Work out the finished part from the listing and answer in its coordinate system (mm). Coordinates: 2 decimals unless noted, no trailing zeros. Loops run counter-clockwise (first coordinate to the right, second up) from the corner with the lowest first, then second, coordinate; pieces in that order, holes last. Notation, with made-up numbers: (41, 48.25) -> (86, 48.25) arc R35 cw to (86, 81.25) -> close; hole circle Ø5 at (60.5, -19). An arc over 180 degrees is marked (long way). Answer as CSV lines item,"result".
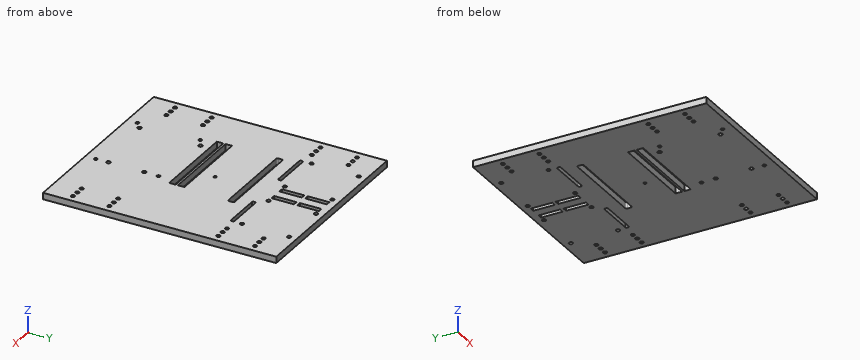
```python
from build123d import *

# Parameters (mm, degrees)
F0_R     = 1.494301
F0_R_2   = 1.356788
F0_R_3   = 1.5875
F0_W     = 66.04
F0_H     = 5.08
F0_W_2   = 3.491225
F0_H_2   = 17.486991
F0_H_3   = 16.910404
F0_R_4   = 1.133922
F1_DEPTH = 5.0038


with BuildPart() as f1:
    # F0 (on Top) → F1 (new body)
    with BuildSketch(Plane.XY):
        Polygon((70.456985, 90.965845), (-70.456985, 90.965845), (-76.806985, 90.965845), (-76.806985, 84.615845), (-76.806985, -84.615845), (-76.806985, -90.965845), (-70.456985, -90.965845), (70.456985, -90.965845), (76.806985, -90.965845), (76.806985, -84.615845), (76.806985, 84.615845), (76.806985, 90.965845), align=None)
        with Locations((-70.824079, -70.982955)):
            Circle(F0_R, mode=Mode.SUBTRACT)
        with Locations((-64.820901, -70.966512)):
            Circle(F0_R, mode=Mode.SUBTRACT)
        with Locations((-58.837254, -70.966512)):
            Circle(F0_R, mode=Mode.SUBTRACT)
        with Locations((-39.865345, -82.879322)):
            Circle(F0_R_2, mode=Mode.SUBTRACT)
        with Locations((-34.309838, -78.185227)):
            Circle(F0_R_3, mode=Mode.SUBTRACT)
        with Locations((-70.834705, -42.482955)):
            Circle(F0_R, mode=Mode.SUBTRACT)
        with Locations((-64.831526, -42.467712)):
            Circle(F0_R, mode=Mode.SUBTRACT)
        with Locations((-58.847879, -42.467712)):
            Circle(F0_R, mode=Mode.SUBTRACT)
        with Locations((-39.865345, -33.888042)):
            Circle(F0_R_2, mode=Mode.SUBTRACT)
        with Locations((-33.039838, -29.925227)):
            Circle(F0_R_3, mode=Mode.SUBTRACT)
        with Locations((-10.337991, -20.430786)):
            Rectangle(F0_W, F0_H, mode=Mode.SUBTRACT)
        with Locations((-10.337991, -13.637)):
            Rectangle(F0_W, F0_H, mode=Mode.SUBTRACT)
        with Locations((18.120408, -82.87932)):
            Circle(F0_R_2, mode=Mode.SUBTRACT)
        with Locations((17.760162, -73.105227)):
            Circle(F0_R_3, mode=Mode.SUBTRACT)
        with Locations((58.837254, -70.966512)):
            Circle(F0_R, mode=Mode.SUBTRACT)
        with Locations((64.820901, -70.966512)):
            Circle(F0_R, mode=Mode.SUBTRACT)
        with Locations((70.824079, -70.982955)):
            Circle(F0_R, mode=Mode.SUBTRACT)
        with Locations((17.760162, -45.165227)):
            Circle(F0_R_3, mode=Mode.SUBTRACT)
        with Locations((18.120408, -33.888042)):
            Circle(F0_R_2, mode=Mode.SUBTRACT)
        with Locations((58.847879, -42.467712)):
            Circle(F0_R, mode=Mode.SUBTRACT)
        with Locations((64.831526, -42.467712)):
            Circle(F0_R, mode=Mode.SUBTRACT)
        with Locations((70.834705, -42.482955)):
            Circle(F0_R, mode=Mode.SUBTRACT)
        with Locations((-70.834705, 42.482955)):
            Circle(F0_R, mode=Mode.SUBTRACT)
        with Locations((-64.831526, 42.467712)):
            Circle(F0_R, mode=Mode.SUBTRACT)
        with Locations((-58.847878, 42.482955)):
            Circle(F0_R, mode=Mode.SUBTRACT)
        with BuildLine():
            ThreePointArc((-48.263557, 40.736089), (-47.935968, 41.52696), (-47.145098, 41.854549))
            Line((-47.145098, 41.854549), (-34.13846, 41.854549))
            Line((-34.13846, 41.854549), (-31.515838, 41.854549))
            Line((-31.515838, 41.854549), (-18.5092, 41.854549))
            ThreePointArc((-18.5092, 41.854549), (-17.718329, 41.52696), (-17.39074, 40.736089))
            Line((-17.39074, 40.736089), (-17.39074, 40.22988))
            ThreePointArc((-17.39074, 40.22988), (-17.718329, 39.43901), (-18.5092, 39.111421))
            Line((-18.5092, 39.111421), (-31.515838, 39.111421))
            Line((-31.515838, 39.111421), (-34.13846, 39.111421))
            Line((-34.13846, 39.111421), (-47.145098, 39.111421))
            ThreePointArc((-47.145098, 39.111421), (-47.935968, 39.43901), (-48.263557, 40.22988))
            Line((-48.263557, 40.22988), (-48.263557, 40.736089))
        make_face(mode=Mode.SUBTRACT)
        with BuildLine():
            Line((23.800469, 23.877405), (-42.239531, 23.877405))
            ThreePointArc((-42.239531, 23.877405), (-43.030401, 24.204994), (-43.357991, 24.995864))
            Line((-43.357991, 24.995864), (-43.357991, 27.672048))
            ThreePointArc((-43.357991, 27.672048), (-43.030401, 28.462918), (-42.239531, 28.790507))
            Line((-42.239531, 28.790507), (15.032583, 28.790507))
            Line((15.032583, 28.790507), (19.658049, 28.790507))
            Line((19.658049, 28.790507), (23.800469, 28.790507))
            ThreePointArc((23.800469, 28.790507), (24.59134, 28.462918), (24.918929, 27.672048))
            Line((24.918929, 27.672048), (24.918929, 24.995864))
            ThreePointArc((24.918929, 24.995864), (24.59134, 24.204994), (23.800469, 23.877405))
        make_face(mode=Mode.SUBTRACT)
        with Locations((-48.263557, 48.184544)):
            Circle(F0_R, mode=Mode.SUBTRACT)
        with Locations((-70.824079, 70.982955)):
            Circle(F0_R, mode=Mode.SUBTRACT)
        with Locations((-64.820901, 70.966512)):
            Circle(F0_R, mode=Mode.SUBTRACT)
        with Locations((-58.837252, 70.981755)):
            Circle(F0_R, mode=Mode.SUBTRACT)
        with Locations((-48.292145, 85.000329)):
            Circle(F0_R, mode=Mode.SUBTRACT)
        with Locations((-11.321435, 48.135974)):
            Circle(F0_R, mode=Mode.SUBTRACT)
        with Locations((-5.441815, 56.879467)):
            Rectangle(F0_W_2, F0_H_2, mode=Mode.SUBTRACT)
        with Locations((-5.441815, 76.696746)):
            Rectangle(F0_W_2, F0_H_3, mode=Mode.SUBTRACT)
        with Locations((-11.321435, 85.151948)):
            Circle(F0_R, mode=Mode.SUBTRACT)
        Circle(F0_R_4, mode=Mode.SUBTRACT)
        with BuildLine():
            Line((31.515838, 39.111421), (18.5092, 39.111421))
            ThreePointArc((18.5092, 39.111421), (17.718329, 39.43901), (17.39074, 40.22988))
            Line((17.39074, 40.22988), (17.39074, 40.736089))
            ThreePointArc((17.39074, 40.736089), (17.718329, 41.52696), (18.5092, 41.854549))
            Line((18.5092, 41.854549), (31.515838, 41.854549))
            Line((31.515838, 41.854549), (34.13846, 41.854549))
            Line((34.13846, 41.854549), (47.145098, 41.854549))
            ThreePointArc((47.145098, 41.854549), (47.935968, 41.52696), (48.263557, 40.736089))
            Line((48.263557, 40.736089), (48.263557, 40.22988))
            ThreePointArc((48.263557, 40.22988), (47.935968, 39.43901), (47.145098, 39.111421))
            Line((47.145098, 39.111421), (34.13846, 39.111421))
            Line((34.13846, 39.111421), (31.515838, 39.111421))
        make_face(mode=Mode.SUBTRACT)
        with Locations((58.847878, 42.482955)):
            Circle(F0_R, mode=Mode.SUBTRACT)
        with Locations((64.831526, 42.467712)):
            Circle(F0_R, mode=Mode.SUBTRACT)
        with Locations((70.834705, 42.482955)):
            Circle(F0_R, mode=Mode.SUBTRACT)
        with Locations((11.321435, 48.135974)):
            Circle(F0_R, mode=Mode.SUBTRACT)
        with Locations((5.441815, 56.879467)):
            Rectangle(F0_W_2, F0_H_2, mode=Mode.SUBTRACT)
        with Locations((5.441815, 76.696746)):
            Rectangle(F0_W_2, F0_H_3, mode=Mode.SUBTRACT)
        with Locations((11.321435, 85.151948)):
            Circle(F0_R, mode=Mode.SUBTRACT)
        with Locations((48.263557, 48.184544)):
            Circle(F0_R, mode=Mode.SUBTRACT)
        with Locations((48.292145, 85.000329)):
            Circle(F0_R, mode=Mode.SUBTRACT)
        with Locations((58.837252, 70.981755)):
            Circle(F0_R, mode=Mode.SUBTRACT)
        with Locations((64.820901, 70.966512)):
            Circle(F0_R, mode=Mode.SUBTRACT)
        with Locations((70.824079, 70.982955)):
            Circle(F0_R, mode=Mode.SUBTRACT)
    extrude(amount=F1_DEPTH)


solid = f1.part
```
(1) Flat-ended cylindrical pins translate along their axes: pin 1 Ø3 at (x, y) = (-28.5, 31.5) entering from -Z; pin 2 Ø2.5 at (x, y) = (48.26, 48.18) entering from -Z. Find the tip coordinate at first contact, or state that the pin passes through.
Computed values:
pin 1,"z = 0"
pin 2,"through"
(2) Consider line 1 along Y through (x, z) = (-3.5, 2.5); line 2 along Y through (x, z) = (-31, 1.3); line 3 along X through (y, z) = (-34, 1). Determine where each line is inside the solid, lowest interval first.
Computed values:
line 1,"-90.97 to -22.97, -17.89 to -16.18, -11.1 to 23.88, 28.79 to 90.97"
line 2,"-90.97 to -22.97, -17.89 to -16.18, -11.1 to 23.88, 28.79 to 39.11, 41.85 to 90.97"
line 3,"-76.81 to -41.22, -38.51 to 16.77, 19.47 to 76.81"
(3) A cutting plane is placed at A-A, the plane x = 28. Write down the section's boundary in (y, z), and give its area (3 significant figures).
Computed values:
outline,"(-90.97, 0) -> (39.11, 0) -> (39.11, 5) -> (-90.97, 5) -> close; (41.85, 0) -> (90.97, 0) -> (90.97, 5) -> (41.85, 5) -> close"
area,"897 mm2"
(4) A cutting plane is placed at B-B, the plane z = 4.1. Count the separate pieces of the cut face and the enclosed holes in it, and give its area (3 significant figures).
Computed values:
separate pieces,"1"
enclosed holes,"50"
area,"26,300 mm2"
